Source: CAD feature listing. Evaluate the final solid. Frame: model axes, mm. A direction names the side the tool comes from. Give positions to 0.01 mm unless a question says otherwise; leave off trailing zeros. Order: outer loops, then holes, each group sorted by start corner. A loop starts at its lowest first (then second) coordinate and runs counter-clockwise, first axis right, second up. Notation, with made-up numbers: M -37.5,27 L -20.5,27 A16 ccw -20.5,38 Z; hole C 66,-6.75 d8. An arc over 180 degrees is marked long. Return JSON: item names as keys, results as strings.
from build123d import *

# Parameters (mm, degrees)
F1_DEPTH = 3
F3_DEPTH = 2
F4_DEPTH = 2


with BuildPart() as f1:
    # F0 (on Top) → F1 (new body)
    with BuildSketch(Plane.XY):
        with BuildLine():
            ThreePointArc((7.5, 1.5), (6.914214, 2.914214), (5.5, 3.5))
            Line((5.5, 3.5), (-5.5, 3.5))
            ThreePointArc((-5.5, 3.5), (-6.914214, 2.914214), (-7.5, 1.5))
            Line((-7.5, 1.5), (-7.5, -1.5))
            ThreePointArc((-7.5, -1.5), (-6.914214, -2.914214), (-5.5, -3.5))
            Line((-5.5, -3.5), (5.5, -3.5))
            ThreePointArc((5.5, -3.5), (6.914214, -2.914214), (7.5, -1.5))
            Line((7.5, -1.5), (7.5, 1.5))
        make_face()
    extrude(amount=F1_DEPTH)

    # F2 (on face) → F3 (join)
    with BuildSketch(Plane.XY.offset(3)):
        with BuildLine():
            ThreePointArc((6, 0.2), (5.414214, 1.614214), (4, 2.2))
            Line((4, 2.2), (-4, 2.2))
            ThreePointArc((-4, 2.2), (-5.414214, 1.614214), (-6, 0.2))
            Line((-6, 0.2), (-6, -0.2))
            ThreePointArc((-6, -0.2), (-5.414214, -1.614214), (-4, -2.2))
            Line((-4, -2.2), (4, -2.2))
            ThreePointArc((4, -2.2), (5.414214, -1.614214), (6, -0.2))
            Line((6, -0.2), (6, 0.2))
        make_face()
    extrude(amount=-F3_DEPTH)

    # F2 (on face) → F4 (cut)
    with BuildSketch(Plane.XY.offset(3)):
        with BuildLine():
            ThreePointArc((6, 0.2), (5.414214, 1.614214), (4, 2.2))
            Line((4, 2.2), (-4, 2.2))
            ThreePointArc((-4, 2.2), (-5.414214, 1.614214), (-6, 0.2))
            Line((-6, 0.2), (-6, -0.2))
            ThreePointArc((-6, -0.2), (-5.414214, -1.614214), (-4, -2.2))
            Line((-4, -2.2), (4, -2.2))
            ThreePointArc((4, -2.2), (5.414214, -1.614214), (6, -0.2))
            Line((6, -0.2), (6, 0.2))
        make_face()
    extrude(amount=-F4_DEPTH, mode=Mode.SUBTRACT)


solid = f1.part
1. Draft query along X for faces 3 (the face through (7.5, 0, 1)), 4 (the face through (0, 0, 0)), 5 (the face through (-6.9, 2.93, 1.48)), 6 (the face through (5.4, -1.63, 2.01)). Return one class per face: pulls with the +X half, pulls with the -X half, needs draft (parallel to the pull), parting line crosses it, or undercut.
Evaluation:
{"face 3": "pulls with the +X half", "face 4": "needs draft", "face 5": "pulls with the -X half", "face 6": "undercut"}
2. Section query B-B (z = 1.6). Return loops of the section in (x, y).
Evaluation:
{"outline": "M -7.5,-1.5 A2 ccw -5.5,-3.5 L 5.5,-3.5 A2 ccw 7.5,-1.5 L 7.5,1.5 A2 ccw 5.5,3.5 L -5.5,3.5 A2 ccw -7.5,1.5 Z; hole M -6,-0.2 A2 ccw -4,-2.2 L 4,-2.2 A2 ccw 6,-0.2 L 6,0.2 A2 ccw 4,2.2 L -4,2.2 A2 ccw -6,0.2 Z"}
3. Set-up query: faces 1 (the face through (0, 3.5, 1)), 2 (the face through (0, 0, 1)). Return all of +Z, -Z, +X, -X, +Y, -Y with unobstructed straight access to the full face (end or side cutting, diameter ignored); none if empty.
Evaluation:
{"face 1": "+Z, -Z, +X, -X, +Y", "face 2": "+Z"}
4. Section query D-D (y = -2.5). Return loops of the section in (x, z), then the cut area to 3 significant figures.
Evaluation:
{"outline": "M -7.23,0 L 7.23,0 L 7.23,3 L -7.23,3 Z", "area": "43.4 mm^2"}
5. Ray query, probe 1 along Y at (x, z) = (3.5, 1.8); probe 2 along Z at (x, y) = (-1.5, 0.5); probe 3 along X at (y, z) = (0, 1.85). Return the intervals inside material, ascending.
Evaluation:
{"probe 1": "y = -3.5 to -2.2, 2.2 to 3.5", "probe 2": "z = 0 to 1", "probe 3": "x = -7.5 to -6, 6 to 7.5"}
6. First-contact query: pin 1 (2 mm diameter, centred on x = -1.5, y = 0, fed in from +Z); pin 2 (4 mm diameter, centred on x = 2.5, y = -0.5, fed in from +Z). Flat tips, straight axial feed; report the tip coordinate or a pass-through.
Evaluation:
{"pin 1": "stops at z = 1", "pin 2": "stops at z = 3"}
7. Section query C-C (z = 0.6). Return loops of the section in (x, y), then the cut area to 3 significant figures.
Evaluation:
{"outline": "M -7.5,-1.5 A2 ccw -5.5,-3.5 L 5.5,-3.5 A2 ccw 7.5,-1.5 L 7.5,1.5 A2 ccw 5.5,3.5 L -5.5,3.5 A2 ccw -7.5,1.5 Z", "area": "102 mm^2"}
8. Section query A-A (x = -0.75). Return loops of the section in (y, z), then the cut area to 3 significant figures.
Evaluation:
{"outline": "M -3.5,0 L 3.5,0 L 3.5,3 L 2.2,3 L 2.2,1 L -2.2,1 L -2.2,3 L -3.5,3 Z", "area": "12.2 mm^2"}
